Geometry: final body of the model. Coordinates: model frame, mm. A direction names the side the tool comes from. Give positions to 0.01 mm unless a question says otherwise; leave off trailing zeros. Write each loop counter-clockwise with the first axis right and the second up, starting at its lowest first coordinate (ties: lowest second). Pieces come first, ordered by that corner, then holes. Notation, with made-up numbers: M 29,32.25 L 84,32.25 A18 ccw 84,40.25 Z; hole C 53,-11 d9. An arc over 180 degrees is marked long. One line per question, with ' | ' between items.
from build123d import *

# Parameters (mm, degrees)
SKETCH1_W           = 102.997
SKETCH1_H           = 94.4372
BOSS_EXTRUDE1_DEPTH = 4.7498
CUT_EXTRUDE2_START  = 4.7498
SKETCH2_W           = 175.9966
SKETCH2_H           = 43.6372
CUT_EXTRUDE2_DEPTH  = 75.780166901
CUT_EXTRUDE6_START  = 47.2186
CUT_EXTRUDE6_DEPTH  = 118.248966901
CUT_EXTRUDE8_START  = -4.7498
SKETCH4_R           = 3.5687
CUT_EXTRUDE8_DEPTH  = 75.780166901
CUT_EXTRUDE10_START = -4.7498
SKETCH5_R           = 3.5687
CUT_EXTRUDE10_DEPTH = 75.780166901


with BuildPart() as part:
    # Sketch1 → Boss-Extrude1 (new, symmetric)
    with BuildSketch(Plane(origin=(0, 0, 0), x_dir=(1, 0, 0), z_dir=(0, 1, 0))):
        Rectangle(SKETCH1_W, SKETCH1_H)
    extrude(amount=BOSS_EXTRUDE1_DEPTH, both=True)

    # Sketch2 → Cut-Extrude2 (cut, through all)
    with BuildSketch(Plane(origin=(0, 0, 0), x_dir=(1, 0, 0), z_dir=(0, 1, 0)).offset(CUT_EXTRUDE2_START)):
        with Locations((-66.4972, 0)):
            Rectangle(SKETCH2_W, SKETCH2_H)
    extrude(amount=-CUT_EXTRUDE2_DEPTH, mode=Mode.SUBTRACT)

    # Sketch3 → Cut-Extrude6 (cut, through all)
    with BuildSketch(Plane.XY.offset(CUT_EXTRUDE6_START)):
        Polygon((-154.4955, -14.2494), (-32.4993, -14.2494), (-60.9981, 14.2494), (-154.4955, 14.2494), align=None)
    extrude(amount=-CUT_EXTRUDE6_DEPTH, mode=Mode.SUBTRACT)

    # Sketch4 → Cut-Extrude8 (cut, through all)
    with BuildSketch(Plane(origin=(0, 0, 0), x_dir=(1, 0, 0), z_dir=(0, 1, 0)).offset(CUT_EXTRUDE8_START)):
        with Locations(Location((-26.8605, -37.211, 0), (0, 0, 270))):
            Circle(SKETCH4_R)
        with Locations(Location((8.0645, -37.211, 0), (0, 0, 270))):
            Circle(SKETCH4_R)
        with Locations(Location((42.9895, -37.211, 0), (0, 0, 270))):
            Circle(SKETCH4_R)
        with Locations(Location((-26.8605, 37.211, 0), (0, 0, 270))):
            Circle(SKETCH4_R)
        with Locations(Location((8.0645, 37.211, 0), (0, 0, 270))):
            Circle(SKETCH4_R)
        with Locations(Location((42.9895, 37.211, 0), (0, 0, 270))):
            Circle(SKETCH4_R)
    extrude(amount=CUT_EXTRUDE8_DEPTH, mode=Mode.SUBTRACT)

    # Sketch5 → Cut-Extrude10 (cut, through all)
    with BuildSketch(Plane(origin=(0, 0, 0), x_dir=(1, 0, 0), z_dir=(0, 1, 0)).offset(CUT_EXTRUDE10_START)):
        with Locations(Location((42.9895, 0, 0), (0, 0, 270))):
            Circle(SKETCH5_R)
    extrude(amount=CUT_EXTRUDE10_DEPTH, mode=Mode.SUBTRACT)


solid = part.part
(1) Draft query along Z for faces 1 (the face through (-46.68, -0.07, -34.34)), 2 (the face through (-1, 0, 47.219)), 3 (the face through (10.5, -0.1, 34.6)). Return one class per face: released by +Z, released by -Z, zero draft, split by the parting line, or undercut.
Working result:
face 1: zero draft | face 2: released by +Z | face 3: undercut
(2) First-contact query: P1, Ø9.5, axis at x = 42.99, z = -37.21, coming from the +Y side; P2, Ø3, axis at y = 1.5, z = -1.5, coming from the -X side; P3, Ø5, axis at y = 1.5, z = -23.5, coming from the -X side. Flat tips, straight axial feed; report the tip coordinate or a pass-through.
Working result:
P1: stops at y = 4.75 | P2: stops at x = 21.5 | P3: stops at x = -50.75
(3) Set-up query: faces 4 (the face through (21.501, 0, 0)), 5 (the face through (-46.68, -0.07, 34.7)). Return all of +Z, -Z, +X, -X, +Y, -Y with unobstructed straight access to the full face (end or side cutting, diameter ignored); none if empty.
Working result:
face 4: -X, +Y, -Y | face 5: +Z, -Z, -X, -Y
(4) Cut plane D-D, the plane z = 38.5. Return loops of the section in (x, y), then the cut area to 3 significant figures.
Working result:
outline: M -51.5,4.75 L -42,-4.75 L -30.19,-4.75 L -30.19,4.75 Z; M -23.53,-4.75 L 4.74,-4.75 L 4.74,4.75 L -23.53,4.75 Z; M 11.39,-4.75 L 39.66,-4.75 L 39.66,4.75 L 11.39,4.75 Z; M 46.32,-4.75 L 51.5,-4.75 L 51.5,4.75 L 46.32,4.75 Z | area: 744 mm^2
(5) Cut plane C-C, the plane y = -3.25. Return loops of the section in (x, z), then the cut area to 3 significant figures.
Working result:
outline: M -43.5,-47.22 L 51.5,-47.22 L 51.5,47.22 L -43.5,47.22 L -43.5,21.82 L 21.5,21.82 L 21.5,-21.82 L -43.5,-21.82 Z; hole C -26.86,-37.21 d7.14; hole C -26.86,37.21 d7.14; hole C 8.06,-37.21 d7.14; hole C 8.06,37.21 d7.14; hole C 42.99,-37.21 d7.14; hole C 42.99,0 d7.14; hole C 42.99,37.21 d7.14 | area: 5,850 mm^2
(6) Cut plane B-B, the plane x = 19.5. Return loops of the section in (y, z), then the cut area to 3 significant figures.
Working result:
outline: M -4.75,-47.22 L 4.75,-47.22 L 4.75,-21.82 L -4.75,-21.82 Z; M -4.75,21.82 L 4.75,21.82 L 4.75,47.22 L -4.75,47.22 Z | area: 483 mm^2
(7) Material intervals for L1, parallel to X at y = 2.75, z = 0; L2, parallel to Z at x = -40, y = -4; L3, parallel to X at y = 3.5, z = 37.5, sorted ascending. Write a range as [from, to].
Working result:
L1: x = [21.5, 39.42], [46.56, 51.5] | L2: z = [-47.22, -21.82], [21.82, 47.22] | L3: x = [-50.25, -30.42], [-23.3, 4.51], [11.62, 39.43], [46.55, 51.5]
(8) Cut plane A-A, the plane z = 0. Return loops of the section in (x, y).
Working result:
outline: M 21.5,-4.75 L 39.42,-4.75 L 39.42,4.75 L 21.5,4.75 Z; M 46.56,-4.75 L 51.5,-4.75 L 51.5,4.75 L 46.56,4.75 Z
